The drawing under review shows one solid part. Ordinate dimensions are in mm from its lowest x, y, z. A direction names the side the tool comes from. Round coordinates to 2 decimals unless told otherwise and drop trailing zeros. Order: outer loops, then holes, each group sorted by start corner. A loop starts at its lowest first (then second) coordinate and runs counter-clockwise, first axis right, second up. Notation, with made-up numbers: M 87,68.25 L 95,68.25 A26 cw 95,96.25 Z; hole C 47,48.25 d7. An arc over 180 degrees is marked long. Answer as a JSON object with one key per item and string values.
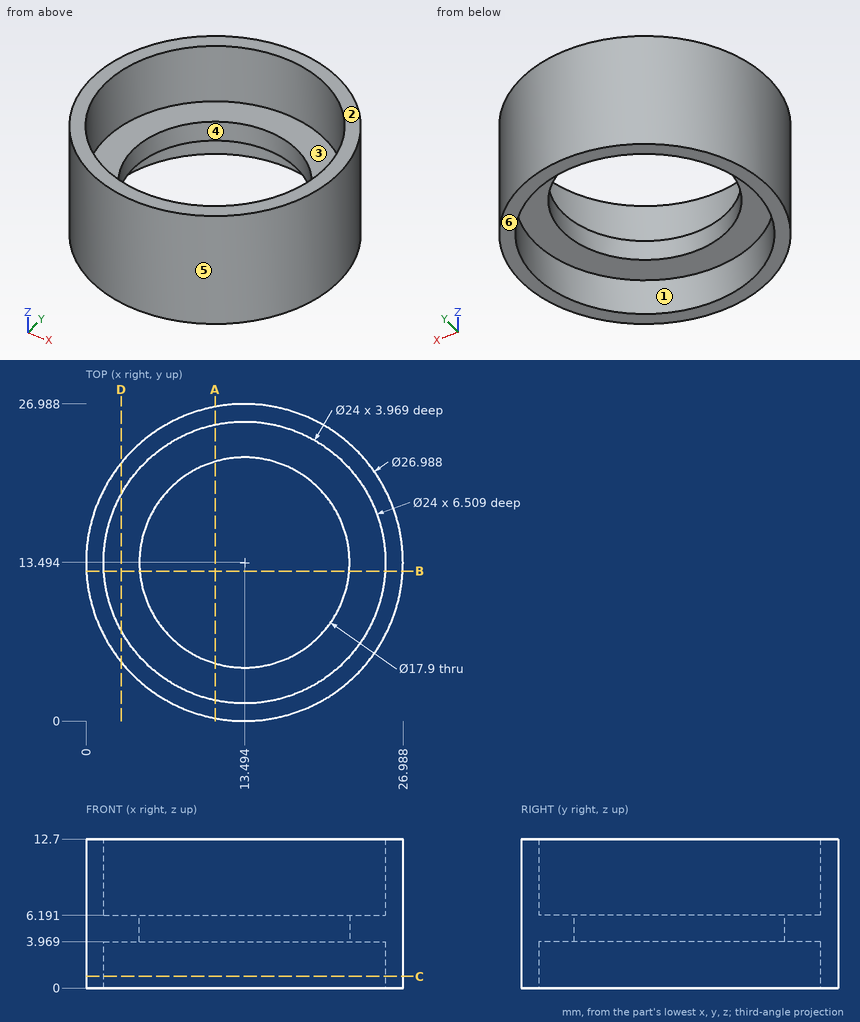
1) For L1, parallel to Z at x = 9, y = 22.25; L2, parallel to Y at x = 14.75, z = 6.5; L3, parallel to Y at x = 13.5, z = 4.5, list the stretches that pass through material, from the lowest coordinate up.
Geometry check:
{"L1": "z = 3.97 to 6.19", "L2": "y = 0.06 to 1.56, 25.43 to 26.93", "L3": "y = 0 to 4.54, 22.44 to 26.99"}
2) Add section C-C on z = 1. State the section outline as (x, y) points.
Geometry check:
{"outline": "C 13.49,13.49 d26.99; hole C 13.49,13.49 d24"}
3) Add section D-D on x = 3. State the section outline as (y, z) points (1 decimal).
Geometry check:
{"outline": "M 5,0 L 7.7,0 L 7.7,4 L 19.3,4 L 19.3,0 L 22,0 L 22,12.7 L 19.3,12.7 L 19.3,6.2 L 7.7,6.2 L 7.7,12.7 L 5,12.7 Z"}
4) Add section A-A on x = 11. State the section outline as (y, z) points (1 decimal).
Geometry check:
{"outline": "M 0.2,0 L 1.8,0 L 1.8,4 L 4.9,4 L 4.9,6.2 L 1.8,6.2 L 1.8,12.7 L 0.2,12.7 Z; M 22.1,4 L 25.2,4 L 25.2,0 L 26.8,0 L 26.8,12.7 L 25.2,12.7 L 25.2,6.2 L 22.1,6.2 Z"}
5) Machinability: for the marked faces 1, 2 and 3, which of the approach directions +Z, -Z, +X, -X, +Y, -Y give a long, thin tool a straight path to every point of the face, cutting with its end or side? Answer none if there is none.
Geometry check:
{"face 1": "-Z", "face 2": "+Z, +X, -X, +Y, -Y", "face 3": "+Z"}
6) Mouldability with a two-part tool opening along Y and no side actions: class the marked faces 4, 5 and 6 as +Y half, -Y half, draft (parallel to the pull), parting line (faces both ways), or undercut.
Geometry check:
{"face 4": "undercut", "face 5": "parting line", "face 6": "draft"}
7) Add section B-B on y = 12.75. State the section outline as (x, z) points (1 decimal).
Geometry check:
{"outline": "M 0,0 L 1.5,0 L 1.5,4 L 4.6,4 L 4.6,6.2 L 1.5,6.2 L 1.5,12.7 L 0,12.7 Z; M 22.4,4 L 25.5,4 L 25.5,0 L 27,0 L 27,12.7 L 25.5,12.7 L 25.5,6.2 L 22.4,6.2 Z"}
8) Insertion check: P1, Ø1.5, axis at x = 4, z = 10.5, coming from the +Y side; P2, Ø1, axis at x = 6, y = 18, coming from the +Z side. Each pin has a flat end and moves straight along its axis. Give the tip position at first contact, or say it passes through.
Geometry check:
{"P1": "stops at y = 23.77", "P2": "stops at z = 6.19"}
